Input: part model. Units: mm. Frame: model coordinates. A direction names the side the tool comes from. Coordinates: 2 decimals unless noted, no trailing zeros. Loops run counter-clockwise (first coordinate to the right, second up) from the corner with the lowest first, then second, coordinate; pieces in that order, holes last. Notation, with made-up numbers: (25.5, 20) -> (45.5, 20) arc R21 cw to (45.5, 55) -> close; hole circle Ø2 at (67.25, 66.5). An arc over 180 degrees is marked (long way). Put each result on its own line as item: value. Start each with the question number.
1) Cut plane D-D (x = 0). State how many separate pieces and enclosed holes the cut face has, plus the area to 3 significant figures.
2) Material intervals for L1, parallel to Y at x = -8.5, z = -243.5; L2, parallel to Y at x = 13.5, z = -248.5, sorted ascending.
3) Cut plane C-C (y = -3.5). Return the cut outline in (x, z).
4) Contact query for flat-ended pins moving along their axis: P1, Ø13.5, axis at x = 0, z = -130, coming from the +Y side; P2, Ø10, axis at x = 18.5, z = -132.5, coming from the -Y side; P3, Ø12, axis at y = 19.5, z = -282, coming from the -X side. Output: stop coordinate, or through.
5) Cut plane A-A (z = -35). Return the cut outline in (x, y), plus the area to 3 significant figures.
6) Cut plane B-B (z = -120). Return the cut outline in (x, y).
7) Set-up query: faces 1 (the flat face through (-22.5, 0, -173)), 2 (the flat face through (25, 0, -173)). Return all of +Z, -Z, +X, -X, +Y, -Y with unobstructed straight access to the full face (end or side cutting, diameter ignored); none if empty.
8) Pull-direction query (Z, two-part tool) for faces 3 (the flat face through (0, 22.5, -173)), 4 (the cylindrical face through (0.183, 23.768, -294.163)); classes: pulls with the +Z half, pulls with the -Z half, needs draft (parallel to the pull), parting line crosses it, or undercut.
from build123d import *

# Parameters (mm, degrees)
SQUARE_TUBE_2_X_2_X_0_25_1_DEPTH = 350
CUT_EXTRUDE1_REACH               = 356.436
SKETCH16_R                       = 7.9375
CUT_EXTRUDE2_REACH               = 356.436
SKETCH18_R                       = 7.9375
CUT_EXTRUDE3_REACH               = 356.436
SKETCH19_R                       = 4.1671875


with BuildPart() as part:
    # Sketch15 → Square tube 2 X 2 X 0.25(1) (new body)
    with BuildSketch(Plane.YX):
        with BuildLine():
            Line((-12.3, -25), (12.3, -25))
            ThreePointArc((12.3, -25), (21.280256121, -21.280256121), (25, -12.3))
            Line((25, -12.3), (25, 12.3))
            ThreePointArc((25, 12.3), (21.280256121, 21.280256121), (12.3, 25))
            Line((12.3, 25), (-12.3, 25))
            ThreePointArc((-12.3, 25), (-21.280256121, 21.280256121), (-25, 12.3))
            Line((-25, 12.3), (-25, -12.3))
            ThreePointArc((-25, -12.3), (-21.280256121, -21.280256121), (-12.3, -25))
        make_face()
        with BuildLine():
            Line((-12.3, -22.5), (12.3, -22.5))
            ThreePointArc((12.3, -22.5), (19.512489168, -19.512489168), (22.5, -12.3))
            Line((22.5, -12.3), (22.5, 12.3))
            ThreePointArc((22.5, 12.3), (19.512489168, 19.512489168), (12.3, 22.5))
            Line((12.3, 22.5), (-12.3, 22.5))
            ThreePointArc((-12.3, 22.5), (-19.512489168, 19.512489168), (-22.5, 12.3))
            Line((-22.5, 12.3), (-22.5, -12.3))
            ThreePointArc((-22.5, -12.3), (-19.512489168, -19.512489168), (-12.3, -22.5))
        make_face(mode=Mode.SUBTRACT)
    extrude(amount=SQUARE_TUBE_2_X_2_X_0_25_1_DEPTH)

    # Cut-Extrude1: up to this face of the body (flat: up to its plane)
    cut_extrude1_end = Plane(part.part.faces().sort_by_distance((25, 0, -175))[0])
    # Sketch16 → Cut-Extrude1 (cut, up to the picked face)
    with BuildSketch(Plane.ZY.offset(25), mode=Mode.PRIVATE) as cut_extrude1_sk1:
        with Locations((-35, 0)):
            Circle(SKETCH16_R)
    cut_extrude1_tool1 = split(extrude(cut_extrude1_sk1.sketch, amount=-CUT_EXTRUDE1_REACH, mode=Mode.PRIVATE), bisect_by=cut_extrude1_end, keep=Keep.BOTH, mode=Mode.PRIVATE)
    add(cut_extrude1_tool1.solids().sort_by(Axis((-25, 0, -35), (1, 0, 0)))[0], mode=Mode.SUBTRACT)

    # Cut-Extrude2: up to this face of the body (flat: up to its plane)
    cut_extrude2_end = Plane(part.part.faces().sort_by_distance((25, 0, -178.294144468))[0])
    # Sketch18 → Cut-Extrude2 (cut, up to the picked face)
    with BuildSketch(Plane.ZY.offset(25), mode=Mode.PRIVATE) as cut_extrude2_sk1:
        with Locations((-315.113369307, 0)):
            Circle(SKETCH18_R)
    cut_extrude2_tool1 = split(extrude(cut_extrude2_sk1.sketch, amount=-CUT_EXTRUDE2_REACH, mode=Mode.PRIVATE), bisect_by=cut_extrude2_end, keep=Keep.BOTH, mode=Mode.PRIVATE)
    add(cut_extrude2_tool1.solids().sort_by(Axis((-25, 0, -315.113369), (1, 0, 0)))[0], mode=Mode.SUBTRACT)

    # Cut-Extrude3: up to this face of the body (flat: up to its plane)
    cut_extrude3_end = Plane(part.part.faces().sort_by_distance((0, -25, -175))[0])
    # Sketch19 → Cut-Extrude3 (cut, up to the picked face)
    with BuildSketch(Plane(origin=(0, 25, 0), x_dir=(-1, 0, 0), z_dir=(0, 1, 0)), mode=Mode.PRIVATE) as cut_extrude3_sk1:
        with Locations(Location((0, -290, 0), (0, 0, 90))):
            Circle(SKETCH19_R)
    cut_extrude3_tool1 = split(extrude(cut_extrude3_sk1.sketch, amount=-CUT_EXTRUDE3_REACH, mode=Mode.PRIVATE), bisect_by=cut_extrude3_end, keep=Keep.BOTH, mode=Mode.PRIVATE)
    # Sketch19 → Cut-Extrude3 (cut, up to the picked face)
    with BuildSketch(Plane(origin=(0, 25, 0), x_dir=(-1, 0, 0), z_dir=(0, 1, 0)), mode=Mode.PRIVATE) as cut_extrude3_sk2:
        with Locations(Location((0, -210, 0), (0, 0, 90))):
            Circle(SKETCH19_R)
    cut_extrude3_tool2 = split(extrude(cut_extrude3_sk2.sketch, amount=-CUT_EXTRUDE3_REACH, mode=Mode.PRIVATE), bisect_by=cut_extrude3_end, keep=Keep.BOTH, mode=Mode.PRIVATE)
    # Sketch19 → Cut-Extrude3 (cut, up to the picked face)
    with BuildSketch(Plane(origin=(0, 25, 0), x_dir=(-1, 0, 0), z_dir=(0, 1, 0)), mode=Mode.PRIVATE) as cut_extrude3_sk3:
        with Locations(Location((0, -130, 0), (0, 0, 90))):
            Circle(SKETCH19_R)
    cut_extrude3_tool3 = split(extrude(cut_extrude3_sk3.sketch, amount=-CUT_EXTRUDE3_REACH, mode=Mode.PRIVATE), bisect_by=cut_extrude3_end, keep=Keep.BOTH, mode=Mode.PRIVATE)
    # Sketch19 → Cut-Extrude3 (cut, up to the picked face)
    with BuildSketch(Plane(origin=(0, 25, 0), x_dir=(-1, 0, 0), z_dir=(0, 1, 0)), mode=Mode.PRIVATE) as cut_extrude3_sk4:
        with Locations(Location((0, -50, 0), (0, 0, 90))):
            Circle(SKETCH19_R)
    cut_extrude3_tool4 = split(extrude(cut_extrude3_sk4.sketch, amount=-CUT_EXTRUDE3_REACH, mode=Mode.PRIVATE), bisect_by=cut_extrude3_end, keep=Keep.BOTH, mode=Mode.PRIVATE)
    add(cut_extrude3_tool1.solids().sort_by(Axis((0, 25, -290), (0, -1, 0)))[0], mode=Mode.SUBTRACT)
    add(cut_extrude3_tool2.solids().sort_by(Axis((0, 25, -210), (0, -1, 0)))[0], mode=Mode.SUBTRACT)
    add(cut_extrude3_tool3.solids().sort_by(Axis((0, 25, -130), (0, -1, 0)))[0], mode=Mode.SUBTRACT)
    add(cut_extrude3_tool4.solids().sort_by(Axis((0, 25, -50), (0, -1, 0)))[0], mode=Mode.SUBTRACT)


solid = part.part
Results found:
1. separate pieces: 10
1. enclosed holes: 0
1. area: 1,580 mm2
2. L1: y = -25 to -22.5, 22.5 to 25
2. L2: y = -24.94 to -22.43, 22.43 to 24.94
3. outline: (-25, -350) -> (-22.5, -350) -> (-22.5, -322.24) -> (-25, -322.24) -> close; (-25, -307.99) -> (-22.5, -307.99) -> (-22.5, -42.12) -> (-25, -42.12) -> close; (-25, -27.88) -> (-22.5, -27.88) -> (-22.5, 0) -> (-25, 0) -> close; (22.5, -350) -> (25, -350) -> (25, -322.24) -> (22.5, -322.24) -> close; (22.5, -307.99) -> (25, -307.99) -> (25, -42.12) -> (22.5, -42.12) -> close; (22.5, -27.88) -> (25, -27.88) -> (25, 0) -> (22.5, 0) -> close
4. P1: stops at y = 25
4. P2: stops at y = -24.94
4. P3: stops at x = -24.94
5. outline: (-25, -12.3) arc R12.7 ccw to (-12.3, -25) -> (12.3, -25) arc R12.7 ccw to (25, -12.3) -> (25, -7.94) -> (22.5, -7.94) -> (22.5, -12.3) arc R10.2 cw to (12.3, -22.5) -> (-12.3, -22.5) arc R10.2 cw to (-22.5, -12.3) -> (-22.5, -7.94) -> (-25, -7.94) -> close; (-25, 7.94) -> (-22.5, 7.94) -> (-22.5, 12.3) arc R10.2 cw to (-12.3, 22.5) -> (12.3, 22.5) arc R10.2 cw to (22.5, 12.3) -> (22.5, 7.94) -> (25, 7.94) -> (25, 12.3) arc R12.7 ccw to (12.3, 25) -> (-12.3, 25) arc R12.7 ccw to (-25, 12.3) -> close
5. area: 346 mm2
6. outline: (-25, -12.3) arc R12.7 ccw to (-12.3, -25) -> (12.3, -25) arc R12.7 ccw to (25, -12.3) -> (25, 12.3) arc R12.7 ccw to (12.3, 25) -> (-12.3, 25) arc R12.7 ccw to (-25, 12.3) -> close; hole (-22.5, -12.3) arc R10.2 ccw to (-12.3, -22.5) -> (12.3, -22.5) arc R10.2 ccw to (22.5, -12.3) -> (22.5, 12.3) arc R10.2 ccw to (12.3, 22.5) -> (-12.3, 22.5) arc R10.2 ccw to (-22.5, 12.3) -> close
7. face 1: +Z, -Z
7. face 2: +Z, -Z, +X, +Y, -Y
8. face 3: needs draft
8. face 4: undercut
